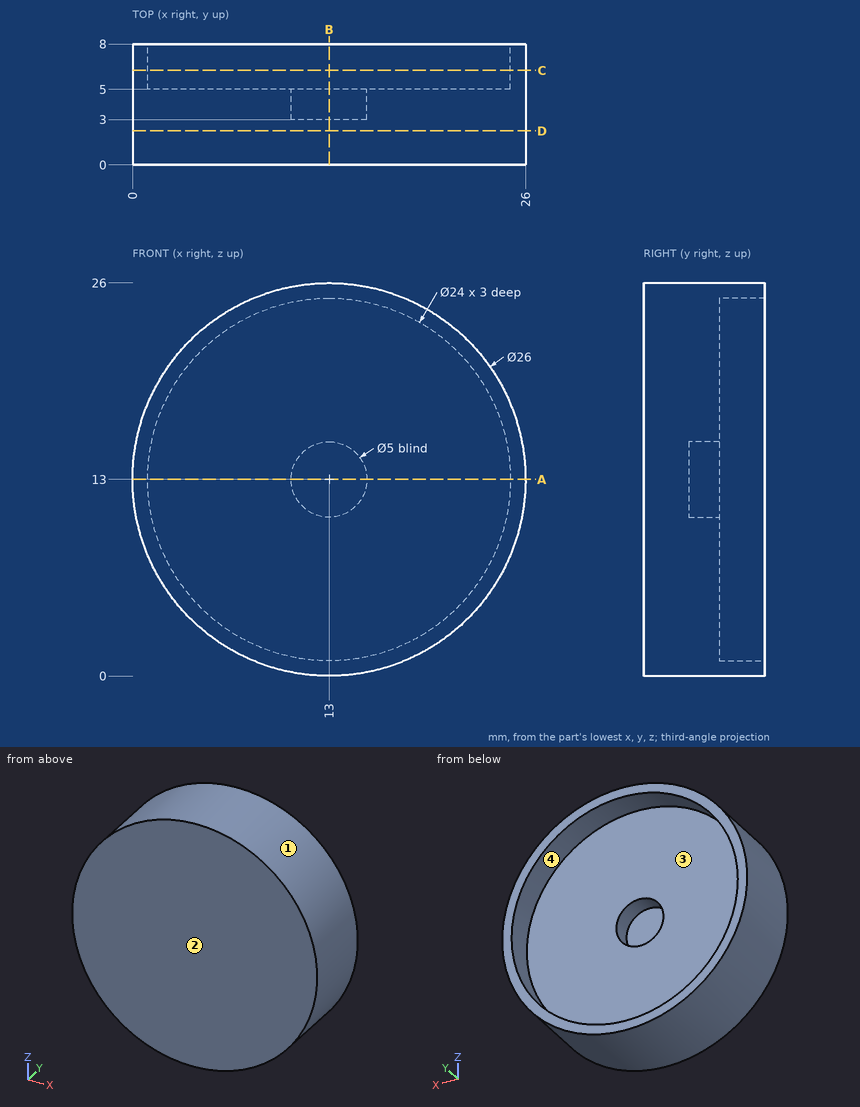
Job drawing, mm, ordinate dimensions from the low corner. One solid piece. Coordinates: 2 decimals unless noted, no trailing zeros. Write each loop counter-clockwise with the first axis right and the second up, starting at its lowest first coordinate (ties: lowest second). Pieces come first, ordered by that corner, then holes. Notation, with made-up numbers: (81.25, -31) - (111.25, -31) arc R13 cw to (111.25, -24) - close; hole circle Ø7 at (76.5, 9). An arc over 180 degrees is marked (long way). Use a Markdown table: item, result. Add a question column.
Item 1: Mould opens along X. For the marked faces 1, 2, 3 and 4 say: pulls with the +X half, pulls with the -X half, needs draft (parallel to the pull), parting line crosses it, or undercut.
Item 2: Flat gauge pins, fed straight in: pin 1 (1.5 mm diameter, centred on x = 16, z = 20, fed in from -Y); pin 2 (3 mm diameter, centred on x = 6.5, y = 2, fed in from +Z); pin 3 (4 mm diameter, centred on x = 12.5, z = 12.5, fed in from +Y); pin 4 (3 mm diameter, centred on y = 4.5, z = 15.5, fed in from -X). Where does each tip first touch, or does it go through?
Item 3: Band-saw the part on B-B, the plane x = 13. Give the cut face in (y, z), and give its area (3 significant figures).
Item 4: Band-saw the part on A-A, the plane z = 13. Give the cut face in (x, y), and give its area (3 significant figures).
Item 5: Drill centre lines: L1, parallel to X at y = 3.45, z = 13; L2, parallel to X at y = 6.4, z = 13; L3, parallel to Y at x = 13, z = 24.75. Where is each one in solid material? Low to high. Write a range as from..to.
Item 6: Band-saw the part on C-C, the plane y = 6.25. Give the cut face in (x, z).
Item 7: Band-saw the part on D-D, the plane y = 2.25. Give the cut face in (x, z), and give its area (3 significant figures).
Numbers:
| question | item | result |
|---|---|---|
| 1 | face 1 | parting line crosses it |
| 1 | face 2 | needs draft |
| 1 | face 3 | undercut |
| 1 | face 4 | undercut |
| 2 | pin 1 | y = 0 |
| 2 | pin 2 | z = 25 |
| 2 | pin 3 | y = 5 |
| 2 | pin 4 | x = 0.04 |
| 3 | outline | (0, 0) - (8, 0) - (8, 1) - (5, 1) - (5, 10.5) - (3, 10.5) - (3, 15.5) - (5, 15.5) - (5, 25) - (8, 25) - (8, 26) - (0, 26) - close |
| 3 | area | 126 mm2 |
| 4 | outline | (0, 0) - (26, 0) - (26, 8) - (25, 8) - (25, 5) - (15.5, 5) - (15.5, 3) - (10.5, 3) - (10.5, 5) - (1, 5) - (1, 8) - (0, 8) - close |
| 4 | area | 126 mm2 |
| 5 | L1 | 0..10.5, 15.5..26 |
| 5 | L2 | 0..1, 25..26 |
| 5 | L3 | 0..5 |
| 6 | outline | circle Ø26 at (13, 13); hole circle Ø24 at (13, 13) |
| 7 | outline | circle Ø26 at (13, 13) |
| 7 | area | 531 mm2 |
